```python
from build123d import *

# Parameters (mm, degrees)
F0_R     = 150
F0_R_2   = 115
F1_DEPTH = 10
F0_R_3   = 140
F0_R_4   = 105
F2_DEPTH = 5


with BuildPart() as f1:
    # F0 (on Top) → F1 (new body)
    with BuildSketch(Plane.XY):
        with BuildLine():
            ThreePointArc((-655.34883, 33.138662), (10.786254, -249.935363), (669.945337, 49.023091))
            Line((669.945337, 49.023091), (0, 650))
            Line((0, 650), (-655.34883, 33.138662))
        make_face()
        Circle(F0_R, mode=Mode.SUBTRACT)
        with Locations((0, 350)):
            Circle(F0_R_2, mode=Mode.SUBTRACT)
    extrude(amount=F1_DEPTH)

    # F0 (on Top) → F2 (join)
    with BuildSketch(Plane.XY):
        Circle(F0_R)
        Circle(F0_R_3, mode=Mode.SUBTRACT)
        with Locations((0, 350)):
            Circle(F0_R_2)
        with Locations((0, 350)):
            Circle(F0_R_4, mode=Mode.SUBTRACT)
    extrude(amount=F2_DEPTH)


solid = f1.part
```
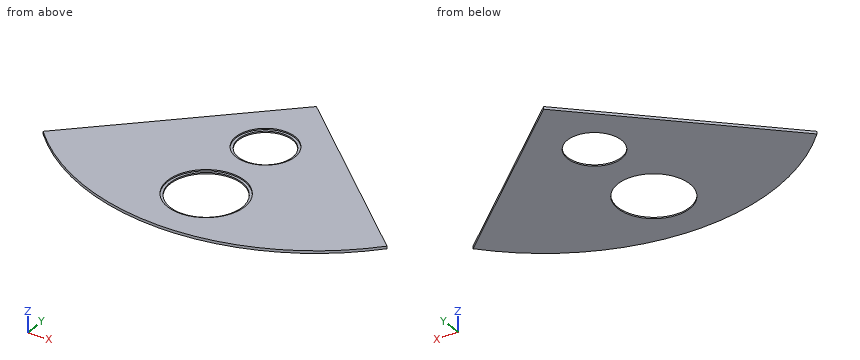
CAD build for the part. Positions are in the model's coordinates, mm. Coordinates: 2 decimals unless noted, no trailing zeros. Order: outer loops, then holes, each group sorted by start corner. A loop starts at its lowest first (then second) coordinate and runs counter-clockwise, first axis right, second up.
(1) Saw through at A-A, the plane z = 6.75. Write the cut outline in (x, y).
Solution:
outline: (-655.35, 33.14) arc R900 ccw to (669.95, 49.02) - (0, 650) - close; hole circle Ø300 at (0, 0); hole circle Ø230 at (0, 350)
(2) Drill centre lines: L1, parallel to Y at x = 0, z = 3.4; L2, parallel to Y at x = 0, z = 8.5; L3, parallel to X at y = 336, z = 8.5. Where is each one in solid material? Low to high.
Solution:
L1: y = -250 to -140, 140 to 245, 455 to 650
L2: y = -250 to -150, 150 to 235, 465 to 650
L3: x = -333.59 to -114.14, 114.14 to 350.03
(3) Saw through at C-C, the plane x = 18. Write the cut outline in (y, z).
Solution:
outline: (-249.82, 0) - (-138.84, 0) - (-138.84, 5) - (-148.92, 5) - (-148.92, 10) - (-249.82, 10) - close; (138.84, 0) - (246.55, 0) - (246.55, 5) - (236.42, 5) - (236.42, 10) - (148.92, 10) - (148.92, 5) - (138.84, 5) - close; (453.45, 0) - (633.85, 0) - (633.85, 10) - (463.58, 10) - (463.58, 5) - (453.45, 5) - close
(4) Pin check, flat tips, straight feed: pin 1 Ø1 at (y, z) = (91, 5.5) entering from -X; pin 2 Ø6 at (x, z) = (478, 3) entering from -Y; pin 3 Ø5 at (y, z) = (-43, 4) entering from -X. Stop position of each tip, or through.
Solution:
pin 1: stops at x = -594.41
pin 2: stops at y = -114.44
pin 3: stops at x = -577.24
(5) Saw through at D-D, the plane y = 0. Write the cut outline in (x, z).
Solution:
outline: (-622.49, 0) - (-140, 0) - (-140, 5) - (-150, 5) - (-150, 10) - (-622.49, 10) - close; (140, 0) - (622.49, 0) - (622.49, 10) - (150, 10) - (150, 5) - (140, 5) - close
(6) Saw through at B-B, the plane y = 350. Write the cut outline in (x, z).
Solution:
outline: (-318.72, 0) - (-105, 0) - (-105, 5) - (-115, 5) - (-115, 10) - (-318.72, 10) - close; (105, 0) - (334.43, 0) - (334.43, 10) - (115, 10) - (115, 5) - (105, 5) - close
